The listing builds one solid part. Answer for the finished solid, in the listing's coordinates (mm). A direction names the side the tool comes from. Give positions to 0.01 mm unless a question says otherwise; leave off trailing zeros. Order: outer loops, then holes, each group sorted by start corner. A loop starts at its lowest first (then second) coordinate and runs counter-clockwise, first axis right, second up. Notation, with made-up numbers: (20, -10) - (59, -10) arc R23 ccw to (59, 10) - close; hole circle Ø11 at (4, -39.75). An arc over 180 degrees is marked (long way). Answer as a JSON object with one key per item and string values. Group by question number.
Q1. Given pin 1 (8 mm diameter, centred on x = 1.5, y = -20, fed in from -Z); pin 2 (3 mm diameter, centred on x = 4, z = -23, fed in from +Y); pin 3 (4 mm diameter, centred on x = -1, y = 2.5, fed in from -Z), each flat-ended and moving along its own axis, determine where each tip first touches the part or whether it passes through.
Q2. A cutting plane is placed at A-A, the plane x = -3. Give the vertices of the cut face in (y, z), and give its area (3 significant figures).
Q3. A cutting plane is placed at B-B, the plane z = -26. Give the vertices of the cut face in (x, y).
Q4. The mould has two halves that part along Y. Classify faces 4 (the face through (6.958, 22.4, 11.4)), 5 (the face through (7.5, 18, -17)), 6 (the face through (0.105, -25.296, -16.128)): released by +Y, released by -Y, zero draft, split by the parting line, or undercut.
Q5. A cutting plane is placed at C-C, the plane x = 5.5. Count the separate pieces of the cut face and the enclosed holes in it, and give its area (3 significant figures).
Q6. For faces 1 (the face through (7.233, 24.357, 5.409)), 2 (the face through (-0.11, 13.57, 3.01)), 3 (the face through (-7.23, 22.44, -11.67)), determine the directions among +Z, -Z, +X, -X, +Y, -Y from which every point of the face is accessible in a straight line to the end or side of a thin tool.
Q7. Consider line 1 (Y direction, x = -7.3, z = 0); line 2 (Y direction, x = -5, z = 12); line 3 (Y direction, x = 6.5, z = -8). Determine where each line is inside the solid, lowest interval first.
from build123d import *


with BuildPart() as part:
    # Sketch1 → Revolve1 (revolve)
    with BuildSketch(Plane.XY, mode=Mode.PRIVATE) as revolve1_sk:
        with BuildLine():
            Line((7.5, 13.9), (-7.5, 13.9))
            Line((-7.5, 13.9), (-7.5, 15.815032431))
            add(Edge.make_bspline(
                [(-7.5, 15.815032431), (-0.221533759, 20.854783747), (-7.5, 24.507708918)],
                knots=[0, 0, 0, 1, 1, 1], degree=2))
            Line((-7.5, 24.507708918), (-7.5, 24.950271606))
            Line((-7.5, 24.950271606), (-6.958076182, 24.950271606))
            Line((-6.958076182, 24.950271606), (-6.958076182, 25.292900784))
            Line((-6.958076182, 25.292900784), (-7.5, 25.292900784))
            Line((-7.5, 25.292900784), (-7.5, 30))
            Line((-7.5, 30), (7.5, 30))
            Line((7.5, 30), (7.5, 25.292900784))
            Line((7.5, 25.292900784), (6.958076182, 25.292900784))
            Line((6.958076182, 25.292900784), (6.958076182, 24.950271606))
            Line((6.958076182, 24.950271606), (7.5, 24.950271606))
            Line((7.5, 24.950271606), (7.5, 24.507708918))
            add(Edge.make_bspline(
                [(7.5, 15.815032431), (0.221533759, 20.854783747), (7.5, 24.507708918)],
                knots=[0, 0, 0, 1, 1, 1], degree=2))
            Line((7.5, 15.815032431), (7.5, 13.9))
        make_face()
    revolve(revolve1_sk.sketch.rotate(Axis((37.422784058, 0, 0), (-1, 0, 0)), 90), axis=Axis((37.422784058, 0, 0), (-1, 0, 0)))


solid = part.part
Reply:
{
 "1": {"pin 1": "stops at z = -25.38", "pin 2": "stops at y = 20.92", "pin 3": "stops at z = -30"},
 "2": {"outline": "circle Ø60 at (0, 0); hole circle Ø27.8 at (0, 0)", "area": "2,220 mm^2"},
 "3": {"outline": "(-7.5, -14.97) - (7.5, -14.97) - (7.5, 14.97) - (-7.5, 14.97) - close"},
 "4": {"face 4": "undercut", "face 5": "zero draft", "face 6": "split by the parting line"},
 "5": {"separate pieces": "2", "enclosed holes": "2", "area": "1,470 mm^2"},
 "6": {"face 1": "+X", "face 2": "+X, -X", "face 3": "-X"},
 "7": {"line 1": "y = -30 to -25.29, -24.95 to -24.41, -15.96 to -13.9, 13.9 to 15.96, 24.41 to 24.95, 25.29 to 30", "line 2": "y = -27.5 to -19.42, -13.37 to -7.01, 7.01 to 13.37, 19.42 to 27.5", "line 3": "y = -28.91 to -22.58, -14.49 to -11.37, 11.37 to 14.49, 22.58 to 28.91"}
}
